Work out the finished part from the listing and answer in its coordinate system (mm). Face numbers are marked on the shaded views. Round coordinates to 2 decimals unless told otherwise and drop trailing zeros. Order: outer loops, then holes, each group sorted by start corner. A loop starts at its lowest first (then second) coordinate and runs counter-clockwise, first axis right, second up. Notation, with made-up numbers: (28.5, -25.5) -> (57.5, -25.5) arc R19 ccw to (57.5, 1.5) -> close; hole circle Ø10 at (57, -1.5). An arc over 180 degrees is marked (long way). Use a Markdown table: item, result. Add a question column.
Item 1: For a pull along Y with two mould halves and no side action, classify the marked faces 1 and 2 as +Y half, -Y half, draft (parallel to the pull), parting line (faces both ways), or undercut.
Item 2: A cutting plane is placed at B-B, the plane y = 11.5. Determine the outline of the cut face in (x, z).
Item 3: Find the intervals of material crossed by L1, parallel to X at y = 34, z = 1; L2, parallel to X at y = 42, z = 1.15; L3, parallel to Y at x = -18, z = 0.95, in increasing order. Write a range as [from, to].
Item 4: A cutting plane is placed at A-A, the plane x = 18. Determine the outline of the cut face in (y, z), plus the area to 3 significant figures.
Item 5: Flat-ended cylindrical pins translate along their axes: P1, Ø1.2, axis at y = 32, z = 1.5, coming from the -X side; P2, Ø1, axis at y = 46.5, z = 2, coming from the -X side; P3, Ø1.5, axis at y = -19, z = 1.5, coming from the +X side; P4, Ø3, axis at x = -14.5, y = 44.5, coming from the +Z side. Find the tip coordinate at first contact, or state that the pin passes through.
Item 6: A cutting plane is placed at C-C, the plane x = -9. Determine the outline of the cut face in (y, z).
from build123d import *

# Parameters (mm, degrees)
F1_DEPTH  = 0.8
F2_R      = 5
F3_R      = 5
F5_DEPTH  = 3
F8_W      = 6
F8_H      = 1.5
F9_DEPTH  = 2
F11_DEPTH = 1.5
F12_DEPTH = 1.5
F6_W      = 6
F6_H      = 1.5
F13_DEPTH = 1
F14_W     = 2
F14_H     = 32
F14_H_2   = 30.375
F15_DEPTH = 2


# Not quite as in the source:
# - an extrude ends at something that could not be found from the text; its depth is read off the source's solid


with BuildPart() as f1:
    # F0 (on Top) → F1 (new body)
    with BuildSketch(Plane.XY):
        with BuildLine():
            Line((20.9010709455, 49.8366734011), (-29.2176790545, 49.8366734011))
            Line((-29.2176790545, 49.8366734011), (-29.2176790545, -31.1633265989))
            Line((-29.2176790545, -31.1633265989), (1.1573209455, -31.1633265989))
            ThreePointArc((1.1573209455, -31.1633265989), (4.122864786, -24.0038704394), (11.2823209455, -21.0383265989))
            Line((11.2823209455, -21.0383265989), (20.9010709455, -21.0383265989))
            Line((20.9010709455, -21.0383265989), (20.9010709455, 49.8366734011))
        make_face()
    extrude(amount=F1_DEPTH)

    # F2
    f2_edges = [f1.edges().sort_by_distance(p)[0] for p in [
        (-29.217679, 49.836673, 0.4),
    ]]
    fillet(f2_edges, radius=F2_R)

    # F3
    f3_edges = [f1.edges().sort_by_distance(p)[0] for p in [
        (-29.217679, -31.163327, 0.4),
    ]]
    fillet(f3_edges, radius=F3_R)

    # F4 (on face) → F5 (join)
    with BuildSketch(Plane.XY.offset(0.8)):
        with BuildLine():
            ThreePointArc((-24.2176790545, 47.8366734011), (-26.338999398, 46.9579937447), (-27.2176790545, 44.8366734011))
            Line((-27.2176790545, 44.8366734011), (-27.2176790545, -26.1633265989))
            ThreePointArc((-27.2176790545, -26.1633265989), (-26.338999398, -28.2846469425), (-24.2176790545, -29.1633265989))
            Line((-24.2176790545, -29.1633265989), (-0.6765930938, -29.1633265989))
            ThreePointArc((-0.6765930938, -29.1633265989), (3.4476025396, -21.9095267037), (11.2823209455, -19.0383265989))
            Line((11.2823209455, -19.0383265989), (18.9010709455, -19.0383265989))
            Line((18.9010709455, -19.0383265989), (18.9010709455, 47.8366734011))
            Line((18.9010709455, 47.8366734011), (-24.2176790545, 47.8366734011))
        make_face()
    extrude(amount=F5_DEPTH)

    # F8 (on face) → F9 (cut)
    with BuildSketch(Plane.YZ.offset(18.9010709455)):
        with Locations((-5.1633265989, 1.55)):
            Rectangle(F8_W, F8_H)
        with Locations((37.8366734011, 1.55)):
            Rectangle(F8_W, F8_H)
    extrude(amount=-F9_DEPTH, mode=Mode.SUBTRACT)

    # F10 (on face) → F11 (cut)
    with BuildSketch(Plane.XY.offset(3.8)):
        with BuildLine():
            Line((-24.2176790545, -18.6633265989), (-27.2176790545, -18.6633265989))
            Line((-27.2176790545, -18.6633265989), (-27.2176790545, -26.1633265989))
            ThreePointArc((-27.2176790545, -26.1633265989), (-26.338999398, -28.2846469425), (-24.2176790545, -29.1633265989))
            Line((-24.2176790545, -29.1633265989), (-0.6765930938, -29.1633265989))
            ThreePointArc((-0.6765930938, -29.1633265989), (3.4476025396, -21.9095267037), (11.2823209455, -19.0383265989))
            Line((11.2823209455, -19.0383265989), (18.9010709455, -19.0383265989))
            Line((18.9010709455, -19.0383265989), (18.9010709455, -11.0383265989))
            Line((18.9010709455, -11.0383265989), (15.9010709455, -11.0383265989))
            Line((15.9010709455, -11.0383265989), (15.9010709455, 0.9616734011))
            Line((15.9010709455, 0.9616734011), (18.9010709455, 0.9616734011))
            Line((18.9010709455, 0.9616734011), (18.9010709455, 31.3366734011))
            Line((18.9010709455, 31.3366734011), (15.9010709455, 31.3366734011))
            Line((15.9010709455, 31.3366734011), (15.9010709455, 43.3366734011))
            Line((15.9010709455, 43.3366734011), (18.9010709455, 43.3366734011))
            Line((18.9010709455, 43.3366734011), (18.9010709455, 47.8366734011))
            Line((18.9010709455, 47.8366734011), (-24.2176790545, 47.8366734011))
            ThreePointArc((-24.2176790545, 47.8366734011), (-26.338999398, 46.9579937447), (-27.2176790545, 44.8366734011))
            Line((-27.2176790545, 44.8366734011), (-27.2176790545, 37.3366734011))
            Line((-27.2176790545, 37.3366734011), (-24.2176790545, 37.3366734011))
            Line((-24.2176790545, 37.3366734011), (-24.2176790545, 25.3366734011))
            Line((-24.2176790545, 25.3366734011), (-27.2176790545, 25.3366734011))
            Line((-27.2176790545, 25.3366734011), (-27.2176790545, -6.6633265989))
            Line((-27.2176790545, -6.6633265989), (-24.2176790545, -6.6633265989))
            Line((-24.2176790545, -6.6633265989), (-24.2176790545, -18.6633265989))
        make_face()
    extrude(amount=-F11_DEPTH, mode=Mode.SUBTRACT)

    # F12 (cut, through all): a face of the model
    f12_faces = [f1.faces().sort_by_distance(p)[0] for p in [
        (-4.8878926555, 10.949585375, 2.3),
    ]]
    extrude(f12_faces, amount=-F12_DEPTH, mode=Mode.SUBTRACT)

    # F6 (on face) → F13 (cut)
    with BuildSketch(Plane(origin=(-27.2176790545, 0, 0), x_dir=(0, -1, 0), z_dir=(-1, 0, 0))):
        with Locations((-31.3366734011, 1.55)):
            Rectangle(F6_W, F6_H)
        with Locations((12.6633265989, 1.55)):
            Rectangle(F6_W, F6_H)
    extrude(amount=-F13_DEPTH, mode=Mode.SUBTRACT)

    # F14 (on face) → F15 (join)
    with BuildSketch(Plane.XY.offset(0.8)):
        with BuildLine():
            Line((-24.2176790545, -29.1633265989), (-0.6765930938, -29.1633265989))
            ThreePointArc((-0.6765930938, -29.1633265989), (3.3030681077, -22.0338606151), (10.9010709455, -19.04432196))
            Line((10.9010709455, -19.04432196), (10.9010709455, -17.0434727244))
            ThreePointArc((10.9010709455, -17.0434727244), (2.6741584042, -19.9644354635), (-2.2644729556, -27.1633265989))
            Line((-2.2644729556, -27.1633265989), (-24.2176790545, -27.1633265989))
            ThreePointArc((-24.2176790545, -27.1633265989), (-24.9247858357, -26.8704333801), (-25.2176790545, -26.1633265989))
            Line((-25.2176790545, -26.1633265989), (-25.2176790545, -18.6633265989))
            Line((-25.2176790545, -18.6633265989), (-27.2176790545, -18.6633265989))
            Line((-27.2176790545, -18.6633265989), (-27.2176790545, -26.1633265989))
            ThreePointArc((-27.2176790545, -26.1633265989), (-26.338999398, -28.2846469425), (-24.2176790545, -29.1633265989))
        make_face()
        Polygon((15.9010709455, -17.0383265989), (15.9010709455, -19.0383265989), (18.9010709455, -19.0383265989), (18.9010709455, -11.0383265989), (16.9010709455, -11.0383265989), (16.9010709455, -17.0383265989), align=None)
        Polygon((18.9010709455, 43.3366734011), (18.9010709455, 47.8366734011), (15.9010709455, 47.8366734011), (15.9010709455, 45.8366734011), (16.9010709455, 45.8366734011), (16.9010709455, 43.3366734011), align=None)
        with BuildLine():
            Line((10.9010709455, 47.8366734011), (-24.2176790545, 47.8366734011))
            ThreePointArc((-24.2176790545, 47.8366734011), (-26.338999398, 46.9579937447), (-27.2176790545, 44.8366734011))
            Line((-27.2176790545, 44.8366734011), (-27.2176790545, 37.3366734011))
            Line((-27.2176790545, 37.3366734011), (-25.2176790545, 37.3366734011))
            Line((-25.2176790545, 37.3366734011), (-25.2176790545, 44.8366734011))
            ThreePointArc((-25.2176790545, 44.8366734011), (-24.9247858357, 45.5437801823), (-24.2176790545, 45.8366734011))
            Line((-24.2176790545, 45.8366734011), (10.9010709455, 45.8366734011))
            Line((10.9010709455, 45.8366734011), (10.9010709455, 47.8366734011))
        make_face()
        with Locations((-26.2176790545, 9.3366734011)):
            Rectangle(F14_W, F14_H)
        with Locations((17.9010709455, 16.1491734011)):
            Rectangle(F14_W, F14_H_2)
    extrude(amount=F15_DEPTH)


solid = f1.part
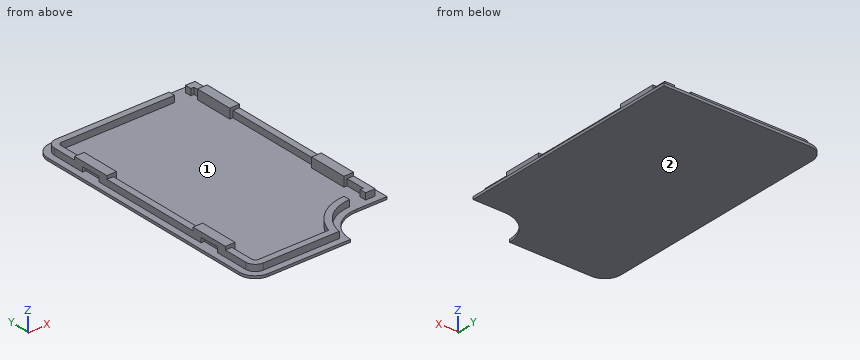
Reported:
| question | item | result |
|---|---|---|
| 1 | face 1 | undercut |
| 1 | face 2 | draft |
| 2 | outline | (-29.22, 0) -> (20.9, 0) -> (20.9, 0.8) -> (18.9, 0.8) -> (18.9, 2.8) -> (16.9, 2.8) -> (16.9, 0.8) -> (-25.22, 0.8) -> (-25.22, 2.8) -> (-27.22, 2.8) -> (-27.22, 0.8) -> (-29.22, 0.8) -> close |
| 3 | L1 | [-26.22, -24.22], [15.9, 18.9] |
| 3 | L2 | [-27.22, -25.22], [15.9, 18.9] |
| 3 | L3 | [-29.16, -27.16], [45.84, 47.84] |
| 4 | outline | (-21.04, 0) -> (49.84, 0) -> (49.84, 0.8) -> (47.84, 0.8) -> (47.84, 2.8) -> (43.34, 2.8) -> (43.34, 3.8) -> (31.34, 3.8) -> (31.34, 2.8) -> (0.96, 2.8) -> (0.96, 3.8) -> (-11.04, 3.8) -> (-11.04, 2.8) -> (-19.04, 2.8) -> (-19.04, 0.8) -> (-21.04, 0.8) -> close; hole (-8.16, 0.8) -> (-2.16, 0.8) -> (-2.16, 2.3) -> (-8.16, 2.3) -> close; hole (34.84, 0.8) -> (40.84, 0.8) -> (40.84, 2.3) -> (34.84, 2.3) -> close |
| 4 | area | 196 mm² |
| 5 | P1 | x = -26.22 |
| 5 | P2 | x = -26.98 |
| 5 | P3 | x = 20.9 |
| 5 | P4 | z = 2.8 |
| 6 | outline | (-31.16, 0) -> (49.84, 0) -> (49.84, 0.8) -> (47.84, 0.8) -> (47.84, 2.8) -> (45.84, 2.8) -> (45.84, 0.8) -> (-27.16, 0.8) -> (-27.16, 2.8) -> (-29.16, 2.8) -> (-29.16, 0.8) -> (-31.16, 0.8) -> close |
